Source: CAD feature listing. Evaluate the final solid. Frame: model axes, mm. Give positions to 0.01 mm unless a question says otherwise; leave off trailing zeros. Write each loop counter-clockwise with the first axis right and the second up, starting at its lowest first coordinate (ties: lowest second). Pieces come first, ordered by that corner, then holes. Notation, with made-up numbers: (0, 27.25) -> (37, 27.25) arc R25 ccw to (37, 45.25) -> close; hole circle Ø8 at (-17, -13.75). An arc over 180 degrees is marked (long way). Write item = value, one per line.
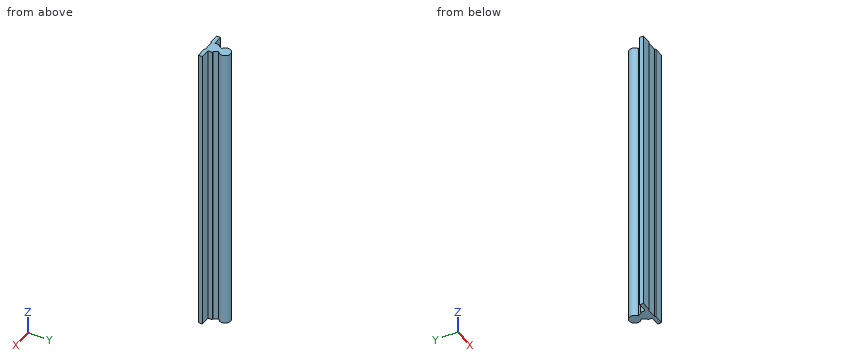
from build123d import *

# Parameters (mm, degrees)
EXTRUDE_1_DEPTH     = 149
SKETCH_2_W          = 10.5
SKETCH_2_H          = 1
CUT_EXTRUDE_1_DEPTH = 300.365635096
CHAMFER_1_SIZE      = 1


with BuildPart() as part:
    # 草图1 → 凸台-拉伸1 (new, symmetric)
    with BuildSketch(Plane.XY):
        with BuildLine():
            Line((-16, 0), (16, 0))
            Line((16, 0), (16, 4))
            Line((16, 4), (6.25, 4))
            Line((6.25, 4), (6.25, 8.5))
            Line((6.25, 8.5), (5.25, 8.5))
            Line((5.25, 8.5), (2.651923789, 13))
            ThreePointArc((2.651923789, 13), (0, 23.659743791), (-2.651923789, 13))
            Line((-2.651923789, 13), (-5.25, 8.5))
            Line((-5.25, 8.5), (-6.25, 8.5))
            Line((-6.25, 8.5), (-6.25, 4))
            Line((-6.25, 4), (-16, 4))
            Line((-16, 4), (-16, 0))
        make_face()
    extrude(amount=EXTRUDE_1_DEPTH, both=True)

    # 草图2 → 切除-拉伸1 (cut, through all)
    with BuildSketch(Plane.XY.offset(149)):
        with Locations((0, 0.5)):
            Rectangle(SKETCH_2_W, SKETCH_2_H)
    extrude(amount=-CUT_EXTRUDE_1_DEPTH, mode=Mode.SUBTRACT)

    # 倒角1
    chamfer_1_edges = [part.edges().sort_by_distance(p)[0] for p in [
        (5.25, 0, 0),
        (-5.25, 0, 0),
    ]]
    chamfer(chamfer_1_edges, length=CHAMFER_1_SIZE - 0.0001)  # a hair under: the kernel refuses the full size


solid = part.part
1) Cut plane C-C (x = 12). Return the cut outline in (y, z), then the cut area to 3 significant figures.
Computed:
outline = (0, -149) -> (4, -149) -> (4, 149) -> (0, 149) -> close
area = 1,190 mm²
2) Contact query for flat-ended pins moving along their axis: pin 1 (5 mm diameter, centred on x = 9.5, z = -55.5, fed in from +Y); pin 2 (0.5 mm diameter, centred on x = -6, z = -5, fed in from +Y); pin 3 (8 mm diameter, centred on y = 21, z = 22, fed in from -X); pin 4 (6 mm diameter, centred on x = -10.5, y = 10, fed in from -Z). Output: stop coordinate, or through.
Computed:
pin_1 = 4
pin_2 = 8.5
pin_3 = -5.66
pin_4 = through
3) Material intervals for L1, parallel to Y at x = -6.5, z = 85; L2, parallel to Y at x = 3, z = 80; L3, parallel to X at y = 13, z = 100.5, sorted ascending.
Computed:
L1 = 0 to 4
L2 = 1 to 12.4, 13.2 to 22.8
L3 = -2.65 to 2.65
4) Cut plane B-B (y = 18). Return the cut outline in (x, z), then the cut area to 3 significant figures.
Computed:
outline = (-5.66, -149) -> (5.66, -149) -> (5.66, 149) -> (-5.66, 149) -> close
area = 3,370 mm²
